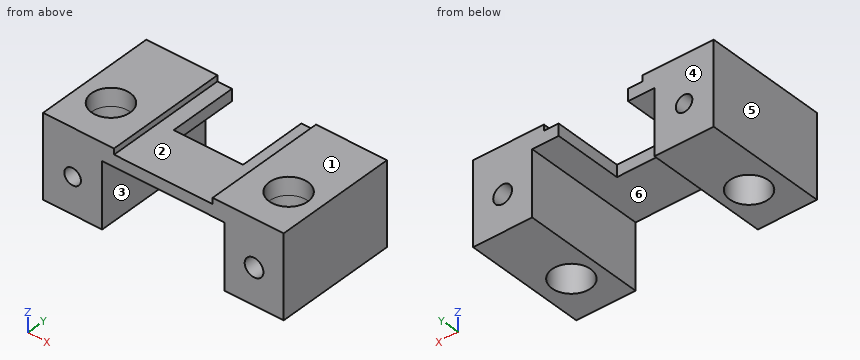
Autodesk Inventor part; units mm, degrees
ref_plane "Work Plane2" through (-20.066, 24.7794, 0) normal (0, 0, 1) x (1, 0, 0)
ref_plane "YZ Plane" through (0, 0, 0) normal (1, 0, 0) x (0, 1, 0)
ref_plane "XZ Plane" through (0, 0, 0) normal (0, 1, 0) x (-1, 0, 0)
ref_plane "Work Plane1" through (0, 37.4307, 11.591) normal (0, 0, 1) x (1, 0, 0)
sketch "Sketch1" plane through (0, 37.4307, 11.591) normal (0, 0, 1) x (1, 0, 0)
  circle A0 centre (0, 0) radius 1.2261 construction
  line L0 (4.85, 4.85) -> (-4.85, 4.85) construction
  line L1 (-4.85, 4.85) -> (-4.85, -4.85) construction
  line L2 (-4.85, -4.85) -> (4.85, -4.85) construction
  line L3 (4.85, -4.85) -> (4.85, 4.85) construction
  line L4 (5.85, 5.85) -> (-5.85, 5.85)
  line L5 (-5.85, 5.85) -> (-5.85, -5.85)
  line L6 (-5.85, -5.85) -> (5.85, -5.85)
  line L7 (5.85, -5.85) -> (5.85, 5.85)
  line L8 (20.32, 25.4487) -> (20.32, -10.6193)
  line L9 (-20.32, -10.6193) -> (-20.32, 25.4487)
  line L10 (5.85, 5.85) -> (20.32, 5.85)
  line L11 (20.32, 5.85) -> (20.32, -5.85)
  line L12 (20.32, -5.85) -> (5.85, -5.85)
  line L13 (5.85, -5.85) -> (5.85, 5.85)
  line L14 (-5.85, 5.85) -> (-20.32, 5.85)
  line L15 (-20.32, 5.85) -> (-20.32, -5.85)
  line L16 (-20.32, -5.85) -> (-5.85, -5.85)
  line L17 (-5.85, -5.85) -> (-5.85, 5.85)
  line L18 (18.034, -12.9053) -> (-18.034, -12.9053)
  line L19 (20.32, -5.85) -> (-20.32, -5.85)
  line L20 (-20.32, -5.85) -> (-20.32, -12.9053)
  line L21 (-20.32, -12.9053) -> (20.32, -12.9053)
  line L22 (20.32, -12.9053) -> (20.32, -5.85)
  point P0 (0, -37.4307)
  dimension "d0" = 1
ref_plane "Work Plane2" through (-20.066, 24.7794, 0) normal (0, 0, 1) x (1, 0, 0)
extrude "Extrusion1" add sketch "Sketch1" against normal blind 3 contours L10 L8 L12 L7 | L5 L16 L9 L14 | L12 L8 L22 L21 L18 L20 L9 L16 L6
sketch "Sketch2" plane through (20.32, 24.5254, 11.591) normal (0, 0, -1) x (-1, 0, 0)
  circle A0 centre (35.32, 5.32) radius 3.0099
  circle A1 centre (5.32, 5.32) radius 3.0099
  circle A2 centre (35.32, 5.32) radius 3.2639
  circle A3 centre (5.32, 5.32) radius 3.2639
extrude "Extrusion2" cut sketch "Sketch2" along normal through all contours A0 | A1 | A2 | A3
sketch "Sketch9" plane through (0, 37.4307, 8.591) normal (0, 0, -1) x (-1, 0, 0)
  line L0 (5.85, -5.85) -> (-5.85, -5.85)
  circle A0 centre (-15, -7.5852) radius 3.2639
  line L1 (-20.32, 5.85) -> (-20.32, -12.9053)
  line L2 (-20.32, -12.9053) -> (20.32, -12.9053)
  line L3 (20.32, -12.9053) -> (20.32, 5.85)
  circle A1 centre (15, -7.5852) radius 3.2639
  line L4 (-5.85, 5.85) -> (-20.32, 5.85)
  line L5 (20.32, 5.85) -> (5.85, 5.85)
  line L6 (5.85, 5.85) -> (5.85, -5.85)
  line L7 (-5.85, -5.85) -> (-5.85, 5.85)
  line L8 (20.32, 5.85) -> (20.32, -12.9053)
  line L9 (20.32, 5.85) -> (5.85, 5.85)
  line L10 (20.32, -12.9053) -> (10.32, -12.9053)
  line L11 (10.32, -12.9053) -> (10.32, 5.85)
  line L12 (10.32, 5.85) -> (20.32, 5.85)
  line L13 (20.32, 5.85) -> (20.32, -12.9053)
  line L14 (-20.32, -12.9053) -> (-10.32, -12.9053)
  line L15 (-10.32, -12.9053) -> (-10.32, 5.85)
  line L16 (-10.32, 5.85) -> (-20.32, 5.85)
  line L17 (-20.32, 5.85) -> (-20.32, -12.9053)
  point P0 (0, -37.4307)
  dimension "d36" = 10
  dimension "d37" = 10
extrude "Extrusion9" add sketch "Sketch9" along normal blind 4 contours L5 L3 L2 L11 | L15 L2 L1 L4
sketch "Sketch10" plane through (-20.32, 24.5254, 11.591) normal (0, -1, 0) x (1, 0, 0)
  line L0 (0, 0) -> (40.64, 0)
  line L1 (0, 0) -> (0, -7)
  line L2 (10, -7) -> (0, -7)
  line L3 (10, -3) -> (10, -7)
  line L4 (30.64, -3) -> (10, -3)
  line L5 (30.64, -3) -> (30.64, -7)
  line L6 (40.64, -7) -> (30.64, -7)
  line L7 (40.64, 0) -> (40.64, -7)
  point P0 (20.32, -11.591)
extrude "Extrusion10" add sketch "Sketch10" along normal blind 2
sketch "Sketch12" plane through (-20.32, 22.5254, 11.591) normal (0, -1, 0) x (1, 0, 0)
  line L0 (40.64, 0) -> (0, 0)
  line L1 (0, 0) -> (0, -7)
  line L2 (0, -7) -> (10, -7)
  line L3 (10, -7) -> (10, -3)
  line L4 (10, -3) -> (30.64, -3)
  line L5 (30.64, -3) -> (30.64, -7)
  line L6 (30.64, -7) -> (40.64, -7)
  line L7 (40.64, -7) -> (40.64, 0)
  line L8 (40.64, 0) -> (26.17, 0)
  line L9 (28.64, 0) -> (12, 0)
  line L10 (12, 0) -> (12, -1)
  line L11 (12, -1) -> (28.64, -1)
  line L12 (28.64, -1) -> (28.64, 0)
  point P0 (20.32, -11.591)
  dimension "d49" = 1
  dimension "d52" = 2
  dimension "d53" = 2
extrude "Extrusion11" cut sketch "Sketch12" against normal through all contours L12 L11 L10 L0
sketch "Sketch13" plane through (0, 37.4307, 4.591) normal (0, 0, -1) x (-1, 0, 0)
  circle A0 centre (15, -7.5852) radius 3.2639
  line L0 (20.32, 5.85) -> (20.32, -14.9053)
  line L1 (20.32, 5.85) -> (10.32, 5.85)
  line L2 (10.32, 5.85) -> (10.32, -14.9053)
  line L3 (20.32, -14.9053) -> (10.32, -14.9053)
  circle A1 centre (-15, -7.5852) radius 3.2639
  line L4 (-10.32, 5.85) -> (-10.32, -14.9053)
  line L5 (-10.32, 5.85) -> (-20.32, 5.85)
  line L6 (-20.32, 5.85) -> (-20.32, -14.9053)
  line L7 (-10.32, -14.9053) -> (-20.32, -14.9053)
  point P0 (0, -37.4307)
extrude "Extrusion12" add sketch "Sketch13" along normal blind 7
sketch "Sketch14" plane through (-10.32, 43.2807, 8.591) normal (0, 1, 0) x (1, 0, 0)
  line L0 (2, -2) -> (4.47, -2)
  line L1 (4.47, -2) -> (4.47, 0)
  line L2 (0, 0) -> (4.47, 0)
  line L3 (0, 0) -> (0, 11)
  line L4 (-10, 11) -> (0, 11)
  line L5 (-10, -3) -> (-10, 11)
  line L6 (2, -3) -> (-10, -3)
  line L7 (2, -3) -> (2, -2)
  line L8 (16.17, -2) -> (18.64, -2)
  line L9 (18.64, -2) -> (18.64, -3)
  line L10 (30.64, -3) -> (18.64, -3)
  line L11 (30.64, -3) -> (30.64, 11)
  line L12 (20.64, 11) -> (30.64, 11)
  line L13 (20.64, 0) -> (20.64, 11)
  line L14 (16.17, 0) -> (20.64, 0)
  line L15 (16.17, -2) -> (16.17, 0)
  line L16 (-7.9439, -3) -> (-7.9439, 11)
  line L17 (-1.4161, -3) -> (-1.4161, 11)
  line L18 (22.0561, -3) -> (22.0561, 11)
  line L19 (28.5839, -3) -> (28.5839, 11)
  circle A0 centre (-5, 4.8877) radius 1.4
  circle A1 centre (25.64, 4.8877) radius 1.5839
  point P0 (10.32, 8.591)
  dimension "d56" = 2.8
extrude "Extrusion13" cut sketch "Sketch14" against normal through all contours A0 | A1
properties part number "20_Adapter_Bluray_KES400_Lens_Thorlabs_v2"
Check sheet for the modelled part. Datum: model origin and axes. Units: mm. Face numbers are marked on the shaded views. A direction names the side the tool comes from. Coordinates: 2 decimals unless noted, no trailing zeros. Order: outer loops, then holes, each group sorted by start corner. A loop starts at its lowest first (then second) coordinate and runs counter-clockwise, first axis right, second up. Notation, with made-up numbers: (-32.5, -17.5) -> (-20.5, -17.5) arc R13 cw to (-20.5, -5.5) -> close; hole circle Ø5 at (67.25, 64.5). An arc over 180 degrees is marked (long way). Write item = value, one per line. Start each with the question number.
1) Cross-section at A-A (y = 40). Enter the section's corners in (x, z).
2) Cross-section at D-D (z = 9.25). Enter the section's corners in (x, y).
3) Cross-section at B-B (z = 6). Enter the section's corners in (x, y).
4) Cross-section at C-C (x = -15.32). State how many separate pieces and enclosed holes the cut face has, then the cut area to 3 significant figures.
5) Mould release check, pull along X, two halves, no side actions. Record for the marked faces 4, 5 and 6: +X half, -X half, draft (parallel to the pull), parting line (faces both ways), or undercut.
6) Go/stop test with flat-tipped pins: P1, Ø10.5, axis at x = 2, y = 31, coming from the -Z side; P2, Ø0.6, axis at x = 2, z = 9.5, coming from the +Y side; P3, Ø1, axis at x = 4.5, y = 33, coming from the -Z side; P4, Ø8.5, axis at x = -1.5, y = 31.5, coming from the +Z side. Record where each tip stops, or that it passes through.
7) Access from +Z, -Z, +X, -X, +Y, -Y to the whole of each face (thin tool, end or side, straight path). Record for the marked faces 1, 2 and 3.
8) Material ranges on L1, parallel to Y at x = -15, z = 0; L2, parallel to X at y = 39.5, z = 9.75; L3, parallel to X at y = 37.75, z = 5.75, recorded low to high.
Ans:
q1.outline = (-20.32, -2.41) -> (-10.32, -2.41) -> (-10.32, 8.59) -> (-5.85, 8.59) -> (-5.85, 10.59) -> (-8.32, 10.59) -> (-8.32, 11.59) -> (-20.32, 11.59) -> close; (5.85, 8.59) -> (10.32, 8.59) -> (10.32, -2.41) -> (20.32, -2.41) -> (20.32, 11.59) -> (8.32, 11.59) -> (8.32, 10.59) -> (5.85, 10.59) -> close; hole circle Ø2.8 at (-15.32, 3.7); hole circle Ø3.17 at (15.32, 3.7)
q2.outline = (-20.32, 22.53) -> (20.32, 22.53) -> (20.32, 43.28) -> (5.85, 43.28) -> (5.85, 31.58) -> (-5.85, 31.58) -> (-5.85, 43.28) -> (-20.32, 43.28) -> close; hole circle Ø6.53 at (-15, 29.85); hole circle Ø6.53 at (15, 29.85)
q3.outline = (-20.32, 22.53) -> (-10.32, 22.53) -> (-10.32, 43.28) -> (-20.32, 43.28) -> close; (10.32, 22.53) -> (20.32, 22.53) -> (20.32, 43.28) -> (10.32, 43.28) -> close; hole circle Ø6.53 at (-15, 29.85); hole circle Ø6.53 at (15, 29.85)
q4.separate_pieces = 4
q4.enclosed_holes = 0
q4.area = 160 mm²
q5.face_4 = draft
q5.face_5 = -X half
q5.face_6 = undercut
q6.P1 = 8.59
q6.P2 = 31.58
q6.P3 = through
q6.P4 = 10.59
q7.face_1 = +Z, +X, -X, +Y, -Y
q7.face_2 = +Z, +Y, -Y
q7.face_3 = -Z, +Y, -Y
q8.L1 = 22.53 to 26.58, 33.11 to 43.28
q8.L2 = -20.32 to -5.85, 5.85 to 20.32
q8.L3 = -20.32 to -10.32, 10.32 to 20.32
